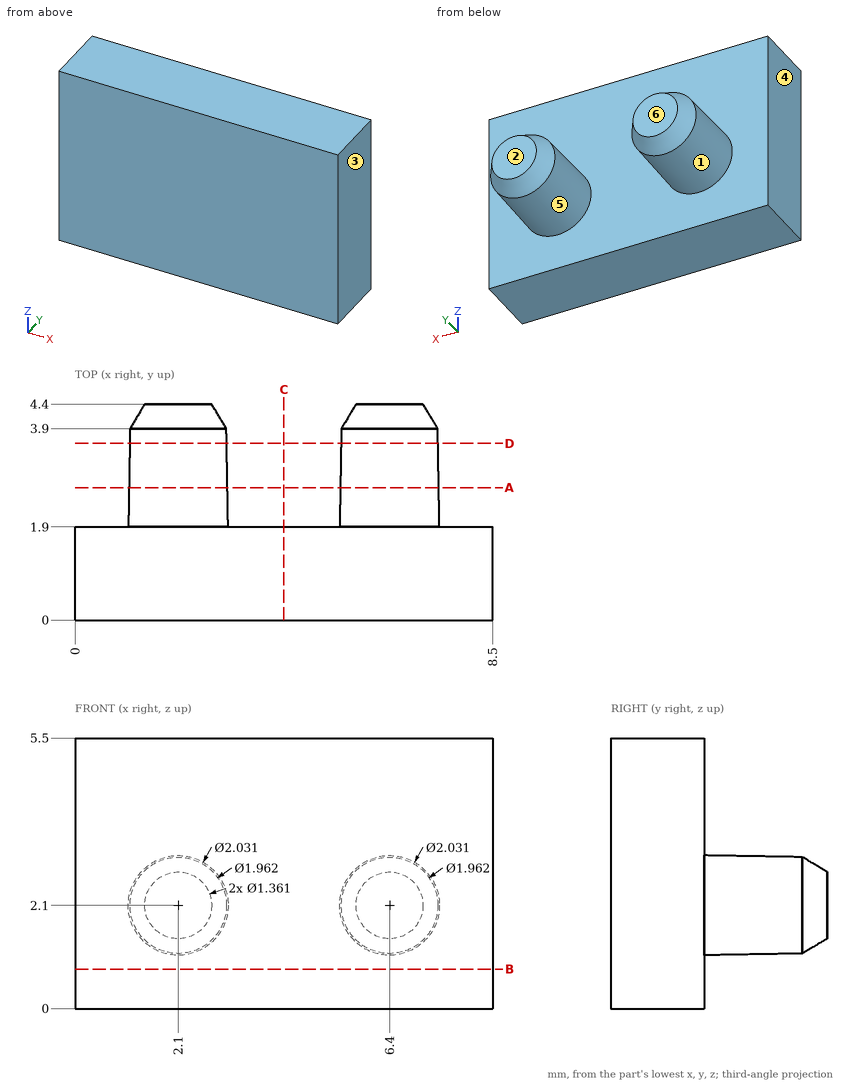
Here's the drawing with two shaded views (mm, measured from the low corner). I have some questions. A direction names the side the tool comes from. Coordinates: 2 decimals unless noted, no trailing zeros. Write each loop counter-clockwise with the first axis right and the second up, starting at its lowest first coordinate (ties: lowest second). Pieces come first, ordered by that corner, then holes.
Item 1: I want a section at C-C on x = 4.25. Write out the boundary of the cut face in (y, z).
Item 2: I want a section at D-D on y = 3.6. Write out the boundary of the cut face in (x, z).
Item 3: Will these pins go through, and if not, where does the flat tip stop? pin 1 (2 mm diameter, centred on y = 3, z = 1, fed in from -X); pin 2 (1.6 mm diameter, centred on x = 2.5, z = 4, fed in from +Y); pin 3 (1 mm diameter, centred on x = 7.5, y = 4, fed in from -Z).
Item 4: If I drill on line 1 (Y direction, x = 2, z = 3.85); line 2 (Z direction, x = 6.5, y = 3.6); line 3 (Z direction, x = 3, y = 3.45) (1 decimal), over which ranges is the centre line in solid material (lowest first)?
Item 5: If we mould it in two halves opening along X, with no side actions, what happens to the marked faces 3, 4, 5 and 6? For each: +X half, -X half, draft (parallel to the pull), parting line (faces both ways), or undercut.
Item 6: I want a section at B-B on z = 0.8. Write out the boundary of the cut face in (x, y).
Item 7: On a 3-axis mill with a long thin cutter (end or side, diameter ignored), from which of +Z, -Z, +X, -X, +Y, -Y can I reach the whole of each face in a straight line? I mean the marked faces 1 and 2. Say none if no direction works.
Item 8: I want a section at A-A on y = 2.7. Write out the boundary of the cut face in (x, z).
Findings below:
1. outline: (0, 0) - (1.9, 0) - (1.9, 5.5) - (0, 5.5) - close
2. outline: circle Ø1.97 at (2.1, 2.1); circle Ø1.97 at (6.4, 2.1)
3. pin 1: stops at x = 1.11
3. pin 2: stops at y = 1.9
3. pin 3: stops at z = 1.33
4. line 1: y = 0 to 1.9
4. line 2: z = 1.12 to 3.08
4. line 3: z = 1.7 to 2.5
5. face 3: +X half
5. face 4: -X half
5. face 5: undercut
5. face 6: draft
6. outline: (0, 0) - (8.5, 0) - (8.5, 1.9) - (0, 1.9) - close
7. face 1: +Y
7. face 2: +Z, -Z, +X, -X, +Y
8. outline: circle Ø2 at (2.1, 2.1); circle Ø2 at (6.4, 2.1)
